Here's how the part is built. I have some questions about the finished solid (model axes, mm). A direction names the side the tool comes from. Round coordinates to 2 decimals unless told otherwise and drop trailing zeros. Write each loop counter-clockwise with the first axis right and the second up, starting at its lowest first coordinate (ties: lowest second). Pieces come first, ordered by that corner, then holes. Notation, with made-up numbers: (-8.75, 28) -> (27.25, 28) arc R34 cw to (27.25, 67) -> close; hole circle Ø5 at (16, 21.25). An arc over 180 degrees is marked (long way). Put each result on its own line as item: value. Start each with the question number.
1) If I drill on line 1 along Z through (x, y) = (-75.5, -1.4); line 2 along X through (y, z) = (-2.2, 33.25); line 3 along X through (y, z) = (-2, 24.25), over which ranges is the centre line in solid material (lowest first)? Write a range as [from, to].
2) Will this pin go through, and if not, where does the flat tip stop? P1, Ø6, axis at x = 36.32, z = 32.37, coming from the -Y side.
3) I want a section at A-A, the plane x = 0. List the corners of the cut face in (y, z) for me.
4) I want a section at B-B, the plane y = -3. List the corners of the cut face in (x, z) for me, then the cut area to 3 significant figures.
5) Which directions (+Z, -Z, +X, -X, +Y, -Y) give clear straight access to the entire face, cutting with the end or side of a thin tool? Please do faces 1 (the flat face through (-82, -2, 24.158)), 2 (the flat face through (-26, 0, 33)).
from build123d import *

# Parameters (mm, degrees)
F0_W     = 158.526307
F0_H     = 30
F0_W_2   = 29.368418
F0_H_2   = 13.894737
F0_R     = 4.878109
F0_R_2   = 4
F0_R_3   = 5
F1_DEPTH = 5


with BuildPart() as f1:
    # F0 (on Front) → F1 (new body)
    with BuildSketch(Plane.XZ):
        with Locations((-25.263152, 32.526316)):
            Rectangle(F0_W, F0_H)
        with Locations((-81.947357, 31.105263)):
            Rectangle(F0_W_2, F0_H_2, mode=Mode.SUBTRACT)
        with Locations((-32.871829, 30.273478)):
            Circle(F0_R, mode=Mode.SUBTRACT)
        with Locations((0, 25.516342)):
            Circle(F0_R_2, mode=Mode.SUBTRACT)
        with Locations((36.315795, 32.368422)):
            Circle(F0_R_3, mode=Mode.SUBTRACT)
    extrude(amount=F1_DEPTH)


solid = f1.part
Findings:
1. line 1: z = [17.53, 24.16], [38.05, 47.53]
1. line 2: x = [-104.53, -96.63], [-67.26, -36.74], [-29.01, 31.39], [41.24, 54]
1. line 3: x = [-104.53, -96.63], [-67.26, -3.79], [3.79, 54]
2. P1: passes through
3. outline: (-5, 17.53) -> (0, 17.53) -> (0, 21.52) -> (-5, 21.52) -> close; (-5, 29.52) -> (0, 29.52) -> (0, 47.53) -> (-5, 47.53) -> close
4. outline: (-104.53, 17.53) -> (54, 17.53) -> (54, 47.53) -> (-104.53, 47.53) -> close; hole (-96.63, 24.16) -> (-67.26, 24.16) -> (-67.26, 38.05) -> (-96.63, 38.05) -> close; hole circle Ø9.76 at (-32.87, 30.27); hole circle Ø8 at (0, 25.52); hole circle Ø10 at (36.32, 32.37)
4. area: 4,140 mm2
5. face 1: +Y, -Y
5. face 2: +Z, -Z, +X, -X, +Y
